Part model, mm, in its own coordinate system. Round coordinates to 2 decimals unless told otherwise and drop trailing zeros. Answer as a JSON object with one key per item and string values. Group by question number.
```python
from build123d import *

# Parameters (mm, degrees)
SKETCH1_R           = 2
BOSS_EXTRUDE1_DEPTH = 1000
SKETCH2_W           = 40
SKETCH2_H           = 20
CUT_EXTRUDE1_DEPTH  = 200


with BuildPart() as part:
    # Sketch1 → Boss-Extrude1 (new body)
    with BuildSketch(Plane.XY):
        Polygon((-5.389620664, 10), (5.389620664, 10), (6.9, 8.2), (4.5, 8.2), (4.5, 6.556171609), (7.151917065, 3.899773171), (9.480384758, 3.899773171), (10, 3.599773171), (10.519615242, 3.899773171), (12.848082935, 3.899773171), (15.5, 6.556171609), (15.5, 8.2), (13.1, 8.2), (14.610379336, 10), (20, 10), (20, 4.610379336), (18.2, 3.1), (18.2, 5.5), (16.556171609, 5.5), (13.9, 2.839339828), (13.9, 0.519615231), (13.599999981, 0), (13.9, -0.519615231), (13.9, -2.839339828), (16.556171609, -5.5), (18.2, -5.5), (18.2, -3.1), (20, -4.610379336), (20, -10), (14.610379336, -10), (13.1, -8.2), (15.5, -8.2), (15.5, -6.556171609), (12.839339828, -3.9), (10.519222362, -3.9), (10, -3.600226829), (9.480777638, -3.9), (7.160660172, -3.9), (4.5, -6.556171609), (4.5, -8.2), (6.9, -8.2), (5.389620664, -10), (-5.389620664, -10), (-6.9, -8.2), (-4.5, -8.2), (-4.5, -6.556171609), (-7.160432959, -3.900226829), (-9.480384758, -3.900226829), (-10, -3.600226829), (-10.519615242, -3.900226829), (-12.839339828, -3.9), (-15.5, -6.556171609), (-15.5, -8.2), (-13.1, -8.2), (-14.610379336, -10), (-20, -10), (-20, -4.610379336), (-18.2, -3.1), (-18.2, -5.5), (-16.556171609, -5.5), (-13.9, -2.839339828), (-13.9, -0.519615231), (-13.599999981, 0), (-13.9, 0.519615231), (-13.9, 2.839339828), (-16.556171609, 5.5), (-18.2, 5.5), (-18.2, 3.1), (-20, 4.610379336), (-20, 10), (-14.610379336, 10), (-13.1, 8.2), (-15.5, 8.2), (-15.5, 6.556171609), (-12.839339828, 3.9), (-10.519615242, 3.899773171), (-10, 3.599773171), (-9.480384758, 3.899773171), (-7.160660172, 3.9), (-4.5, 6.556171609), (-4.5, 8.2), (-6.9, 8.2), align=None)
        with Locations((-10, 0)):
            Circle(SKETCH1_R, mode=Mode.SUBTRACT)
        with Locations((10, 0)):
            Circle(SKETCH1_R, mode=Mode.SUBTRACT)
        Polygon((-6.1, -2.839339828), (-2.376887287, -6.556171609), (-2.376887287, -8.2), (2.376887287, -8.2), (2.376887287, -6.556171609), (6.1, -2.839339828), (6.1, 2.839339828), (2.383168219, 6.556171609), (2.383168219, 8.2), (-2.383168219, 8.2), (-2.383168219, 6.556171609), (-6.1, 2.839339828), align=None, mode=Mode.SUBTRACT)
    extrude(amount=BOSS_EXTRUDE1_DEPTH)

    # Sketch2 → Cut-Extrude1 (cut)
    with BuildSketch(Plane.XY.offset(1000)):
        Rectangle(SKETCH2_W, SKETCH2_H)
    extrude(amount=-CUT_EXTRUDE1_DEPTH, mode=Mode.SUBTRACT)


solid = part.part
```
Q1. Wall check: line 1 (X direction, y = 0, z = 297.5); line 2 (X direction, y = 6.5, z = 402.5); line 3 (X direction, y = 9, z = 581). Give the ranges that are in metal, low to high. Write a range as [from, to].
Q2. Drop flat-ended pins along their axis: pin 1 Ø3 at (x, z) = (-11, 415.5) entering from -Y; pin 2 Ø1.9 at (x, z) = (-12, 593.5) entering from -Y. Give the stop position or say it passes through.
Q3. Band-saw the part on A-A (z = 138). Count the separate pieces of the cut face and the enclosed holes in it, plus the area to 3 significant figures.
Completed:
{
 "1": {"line 1": "[-13.6, -12], [-8, -6.1], [6.1, 8], [12, 13.6]", "line 2": "[-20, -15.44], [-4.56, -2.44], [2.44, 4.56], [15.44, 20]", "line 3": "[-20, -13.77], [-6.23, 6.23], [13.77, 20]"},
 "2": {"pin 1": "y = -3.9", "pin 2": "y = -4.01"},
 "3": {"separate pieces": "1", "enclosed holes": "3", "area": "301 mm2"}
}
